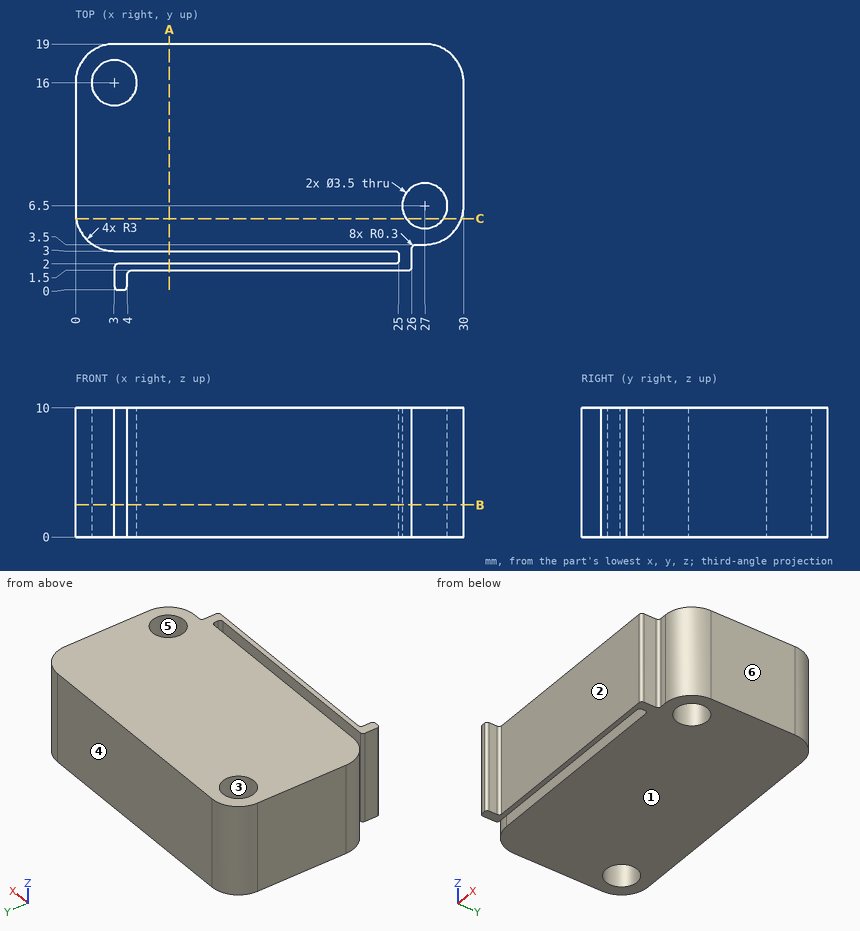
Job drawing, mm, ordinate dimensions from the low corner. One solid piece. A direction names the side the tool comes from. Give positions to 0.01 mm unless a question says otherwise; leave off trailing zeros. Loops run counter-clockwise (first coordinate to the right, second up) from the corner with the lowest first, then second, coordinate; pieces in that order, holes last.
Item 1: Slice it at B-B, the plane z = 2.5. List the corners of the cut face in (x, y), and give its area (3 significant figures).
Answers follow:
outline: (0, 6) arc R3 ccw to (3, 3) - (24.7, 3) arc R0.3 cw to (25, 2.7) - (25, 2.3) arc R0.3 cw to (24.7, 2) - (3.3, 2) arc R0.3 ccw to (3, 1.7) - (3, 0.3) arc R0.3 ccw to (3.3, 0) - (3.7, 0) arc R0.3 ccw to (4, 0.3) - (4, 1.2) arc R0.3 cw to (4.3, 1.5) - (25.7, 1.5) arc R0.3 ccw to (26, 1.8) - (26, 3.2) arc R0.3 cw to (26.3, 3.5) - (27, 3.5) arc R3 ccw to (30, 6.5) - (30, 16) arc R3 ccw to (27, 19) - (3, 19) arc R3 ccw to (0, 16) - close; hole circle Ø3.5 at (3, 16); hole circle Ø3.5 at (27, 6.5)
area: 465 mm2
Item 2: Pull direction X, two halves, no side cores. Call the marked faces 3, 4, 5 and 6: released by +X, released by -X, zero draft, split by the parting line, or undercut.
Answers follow:
face 3: undercut
face 4: zero draft
face 5: undercut
face 6: released by +X
Item 3: Slice it at A-A, the plane x = 7.25. List the corners of the cut face in (y, z), and give its area (3 significant figures).
Answers follow:
outline: (1.5, 0) - (2, 0) - (2, 10) - (1.5, 10) - close; (3, 0) - (19, 0) - (19, 10) - (3, 10) - close
area: 165 mm2
Item 4: Which spindle directions (+Z, -Z, +X, -X, +Y, -Y) get a long thin tool onto all of the face, cutting with end or side? Do the marked faces 1 and 2. Say none if no direction does.
Answers follow:
face 1: -Z, +X, -X, +Y, -Y
face 2: +Z, -Z, +X, -Y
Item 5: Flat gauge pins, fed straight in: pin 1 (1.1 mm diameter, centred on y = 1, z = 4, fed in from -X); pin 2 (2 mm diameter, centred on x = 27, y = 6.5, fed in from -Z); pin 3 (0.7 mm diameter, centred on y = 3, z = 4.5, fed in from +X); pin 4 (5 mm diameter, centred on x = 18.5, z = 7.5, fed in from -Y). Where does each tip first touch, or does it go through?
Answers follow:
pin 1: stops at x = 3
pin 2: passes through
pin 3: stops at x = 26.04
pin 4: stops at y = 1.5
Item 6: Slice it at C-C, the plane y = 5.5. List the corners of the cut face in (x, z), and give its area (3 significant figures).
Answers follow:
outline: (0.04, 0) - (25.56, 0) - (25.56, 10) - (0.04, 10) - close; (28.44, 0) - (29.83, 0) - (29.83, 10) - (28.44, 10) - close
area: 269 mm2
Item 7: Drill centre lines: line 1 (Y direction, x = 18.5, z = 3); line 2 (Y direction, x = 27, z = 2); line 3 (X direction, y = 15.75, z = 0.5). Where is each one in solid material? Low to high.
Answers follow:
line 1: y = 1.5 to 2, 3 to 19
line 2: y = 3.5 to 4.75, 8.25 to 19
line 3: x = 0 to 1.27, 4.73 to 30
